Here's how the part is built. I have some questions about the finished solid (model axes, mm). A direction names the side the tool comes from. Give positions to 0.01 mm unless a question says otherwise; leave off trailing zeros. Write each loop counter-clockwise with the first axis right and the second up, starting at its lowest first coordinate (ties: lowest second). Pieces come first, ordered by that corner, then holes. Notation, with made-up numbers: (42, 23.5) -> (67, 23.5) arc R25 ccw to (67, 35.5) -> close; hole circle Ø1 at (-24, 17). An arc over 180 degrees is marked (long way). Return JSON: item names as keys, results as strings.
Autodesk Inventor part; units mm, degrees
ref_plane "YZ Plane" through (0, 0, 0) normal (1, 0, 0) x (0, 1, 0)
ref_plane "XZ Plane" through (0, 0, 0) normal (0, 1, 0) x (-1, 0, 0)
ref_plane "XY Plane" through (0, 0, 0) normal (0, 0, 1) x (1, 0, 0)
sketch "草圖1" plane through (0, 0, 0) normal (0, 1, 0) x (-1, 0, 0)
  line L0 (12.2, 0) -> (-12.2, 0)
  line L1 (-12.2, 0) -> (-12.2, -53.6)
  line L2 (-12.2, -53.6) -> (12.2, -53.6)
  line L3 (12.2, -53.6) -> (12.2, 0)
  line L4 (2, 0) -> (-2, 0)
  line L5 (-2, 0) -> (-2, 12)
  line L6 (-2, 12) -> (2, 12)
  line L7 (2, 12) -> (2, 0)
  line L8 (3.5, 0) -> (-3.5, 0)
  line L9 (-3.5, 0) -> (-3.5, 2.3)
  line L10 (-3.5, 2.3) -> (3.5, 2.3)
  line L11 (3.5, 2.3) -> (3.5, 0)
  line L12 (2, 4) -> (-2, 4)
  line L13 (8.5, 0) -> (8.5, -53.6)
  line L14 (-8.5, 0) -> (-8.5, -53.6)
  line L15 (0, 0) -> (0, -53.6)
  line L16 (0, 0) -> (0, 12)
  point P0 (-8.5, -26.8)
  point P1 (0, 2.3)
  point P2 (2, 2.3)
  dimension "d1" = 8
  dimension "d2" = 9.7
  dimension "d4" = 17
  dimension "d5" = 24.4
  dimension "d6" = 53.6
  dimension "d7" = 3.7
  dimension "d8" = 4
  dimension "d9" = 7
  dimension "d10" = 2.3
revolve "迴轉1" add sketch "草圖1" angle 360 about axis through (0, 0, 0) along (0, 0, -1) contours L3 L2 L13 L0 | L13 L2 L15 L0 | L0 L7 L10 L11
sketch "草圖4" plane through (0, 0, 0) normal (0, 0, 1) x (1, 0, 0)
  circle A0 centre (0, 0) radius 8.5
  circle A1 centre (0, 8.5) radius 1.4
  circle A2 centre (0, -8.5) radius 1.4
  dimension "d21" = 17
  dimension "d22" = 2.8
  dimension "d23" = 2.8
extrude "擠出3" cut sketch "草圖4" against normal blind 3 contours A1 A0 | A0 A1 | A2 A0 | A0 A2
properties part number "馬達" material "鋁合金 6061"
1. Suppose I cut it at C-C, the plane z = -48. List the corners of the cut face in (x, y) for me, and give its area (3 significant figures).
Taken from the geometry:
{"outline": "circle Ø24.4 at (0, 0)", "area": "468 mm²"}
2. For pin 1 Ø3 at (x, y) = (-0.5, 8.5) entering from +Z; pin 2 Ø1 at (x, z) = (5.5, -36) entering from +Y; pin 3 Ø1.5 at (x, z) = (-1, -46.5) entering from +Y, each with a flat end and sliding along its axis, tell me the tip position at first contact or that it passes through.
Taken from the geometry:
{"pin 1": "stops at z = 0", "pin 2": "stops at y = 11.13", "pin 3": "stops at y = 12.2"}
3. If I drill on line 1 (Y direction, x = 0, z = -1.7); line 2 (Y direction, x = 0, z = 1.15); line 3 (Z direction, x = 9.25, y = -1), over which ranges is the centre line in solid material (lowest first)? Write a range as [from, to].
Taken from the geometry:
{"line 1": "y = [-12.2, -9.9], [-7.1, 7.1], [9.9, 12.2]", "line 2": "y = [-3.5, -2], [2, 3.5]", "line 3": "z = [-53.6, 0]"}
4. Suppose I cut it at D-D, the plane y = 8.5. List the corners of the cut face in (x, z) for me, and give its area (3 significant figures).
Taken from the geometry:
{"outline": "(-8.75, -53.6) -> (8.75, -53.6) -> (8.75, 0) -> (1.4, 0) -> (1.4, -3) -> (-1.4, -3) -> (-1.4, 0) -> (-8.75, 0) -> close", "area": "930 mm²"}
5. Which directions (+Z, -Z, +X, -X, +Y, -Y) give clear straight access to the entire face, cutting with the end or side of a thin tool? Please do faces 5 (the face through (12.19, -0.54, -26.42)), 6 (the face through (-0.303, -9.867, -1.479)).
Taken from the geometry:
{"face 5": "+Z, -Z", "face 6": "+Z"}
6. Suppose I cut it at B-B, the plane y = 0. List the corners of the cut face in (x, z) for me, and give its area (3 significant figures).
Taken from the geometry:
{"outline": "(-12.2, -53.6) -> (12.2, -53.6) -> (12.2, 0) -> (3.5, 0) -> (3.5, 2.3) -> (2, 2.3) -> (2, 0) -> (-2, 0) -> (-2, 2.3) -> (-3.5, 2.3) -> (-3.5, 0) -> (-12.2, 0) -> close", "area": "1,310 mm²"}
7. Suppose I cut it at A-A, the plane x = 0. List the corners of the cut face in (y, z) for me, and give its area (3 significant figures).
Taken from the geometry:
{"outline": "(-12.2, -53.6) -> (12.2, -53.6) -> (12.2, 0) -> (9.9, 0) -> (9.9, -3) -> (7.1, -3) -> (7.1, 0) -> (3.5, 0) -> (3.5, 2.3) -> (2, 2.3) -> (2, 0) -> (-2, 0) -> (-2, 2.3) -> (-3.5, 2.3) -> (-3.5, 0) -> (-7.1, 0) -> (-7.1, -3) -> (-9.9, -3) -> (-9.9, 0) -> (-12.2, 0) -> close", "area": "1,300 mm²"}
8. If we mould it in two halves opening along X, with no side actions, what happens to faces 1 (the face through (0, 9, -3)), 2 (the face through (-3, -3, 0)), 3 (the face through (-3.233, -1.341, 1.134)), 4 (the face through (0, -2, 1))? For each: released by +X, released by -X, zero draft, split by the parting line, or undercut.
Taken from the geometry:
{"face 1": "undercut", "face 2": "zero draft", "face 3": "split by the parting line", "face 4": "undercut"}
